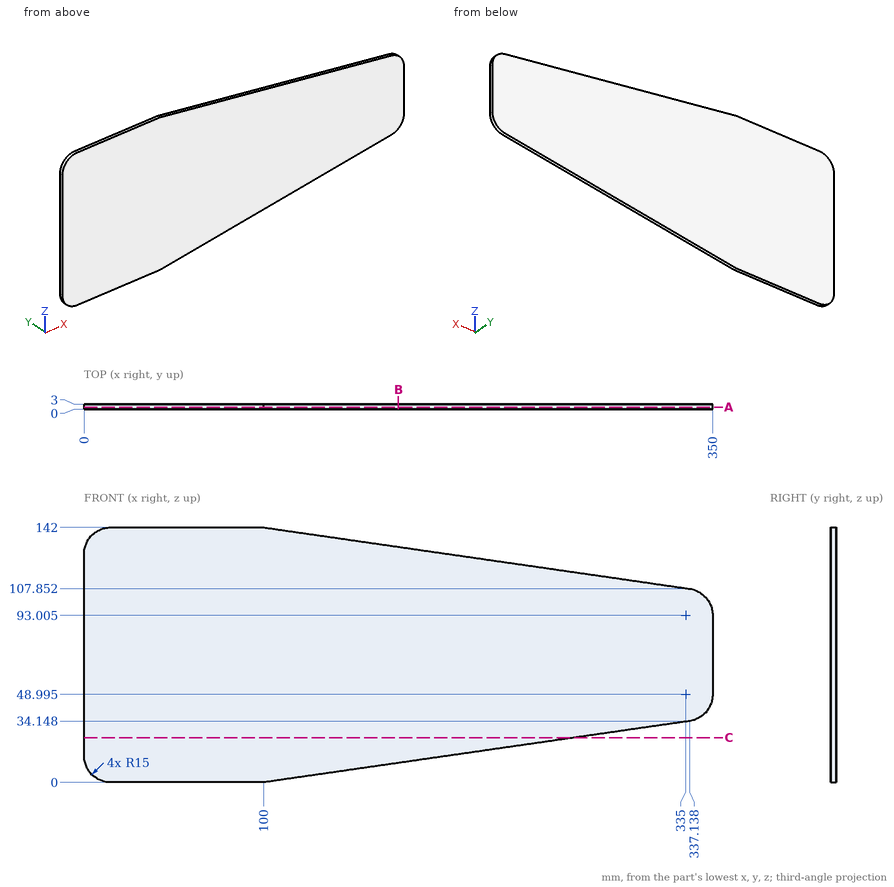
Print and shaded views of the part. All mm, measured from the part's lowest x, y and z. Coordinates: 2 decimals unless noted, no trailing zeros. Loops run counter-clockwise (first coordinate to the right, second up) from the corner with the lowest first, then second, coordinate; pieces in that order, holes last. Notation, with made-up numbers: M 16.25,74.25 L 24.25,74.25 A23 cw 24.25,103.25 Z; hole C 57,-20 d11. An arc over 180 degrees is marked long. Use a Markdown table: item, result. Add a question column.
Q1. Cut at A-A (y = 1.2). Write the cut outline in (x, z) (1 decimal).
Q2. Cut at C-C (z = 25). Write the cut outline in (x, y).
Q3. Probe L1, parallel to Z at x = 182, y = 0.9; L2, parallel to Z at x = 167.5, y = 2; L3, parallel to X at y = 0.45, z = 101.5. List the from-to ranges inside material, lowest first.
Q4. Cut at B-B (x = 175). Write the cut outline in (y, z).
Q5. Pin check, flat tip, straight feed: P1, Ø6, axis at x = 67, z = 88, coming from the -Y side. Stop position of the tip, or through.
Worked out:
| question | item | result |
|---|---|---|
| 1 | outline | M 0,15 A15 ccw 15,0 L 100,0 L 337.1,34.1 A15 ccw 350,49 L 350,93 A15 ccw 337.1,107.9 L 100,142 L 15,142 A15 ccw 0,127 Z |
| 2 | outline | M 0,0 L 273.61,0 L 273.61,3 L 0,3 Z |
| 3 | L1 | z = 11.81 to 130.19 |
| 3 | L2 | z = 9.72 to 132.28 |
| 3 | L3 | x = 0 to 347.36 |
| 4 | outline | M 0,10.8 L 3,10.8 L 3,131.2 L 0,131.2 Z |
| 5 | P1 | stops at y = 0 |
